The drawing under review shows one solid part. Ordinate dimensions are in mm from its lowest x, y, z. Give positions to 0.01 mm unless a question says otherwise; leave off trailing zeros. Order: outer loops, then holes, each group sorted by start corner. A loop starts at its lowest first (then second) coordinate and runs counter-clockwise, first axis right, second up. Notation, with made-up numbers: (22.25, 77) - (74.25, 77) arc R3 ccw to (74.25, 82) - close; hole circle Ø10 at (56.5, 61). An arc over 180 degrees is marked (long way). Use CSV: the item, a comma, the result in double quotes. Start each with the question number.
1. For pin 1 (2 mm diameter, centred on x = 86, y = 5, fed in from -Z); pin 2 (3 mm diameter, centred on x = 90, z = 9.5, fed in from -Y); pin 3 (8 mm diameter, centred on x = 62, z = 4, fed in from +Y), all flat-tipped, find the tip position at first contact; note any pin that passes through.
2. Take a section at C-C, the plane x = 7. State the section outline as (y, z) points.
3. Take a section at B-B, the plane z = 7. State the section outline as (x, y) points.
4. To check wall thickness, follow line 1 (X direction, y = 3, z = 7); line 2 (X direction, y = 4.5, z = 8.25); line 3 (Y direction, x = 43, z = 7). State the ranges of each line that lie inside material, in increasing order. Write a range as [from, to].
5. Take a section at A-A, the plane y = 3.5. State the section outline as (x, z) points.
6. Take a section at D-D, the plane x = 84. State the section outline as (y, z) points.
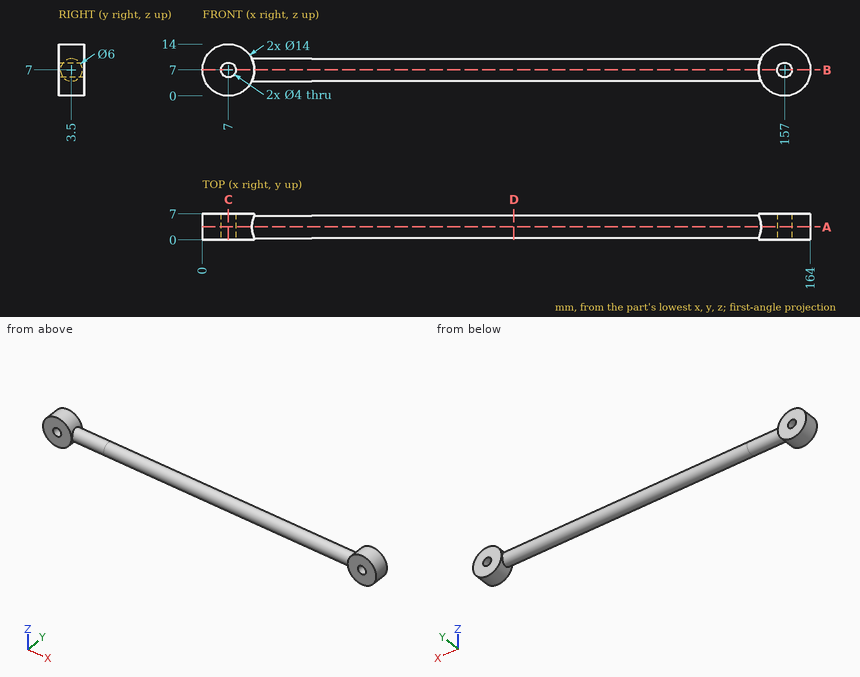
Determined:
1,pin 1,"stops at z = 4.04"
1,pin 2,"stops at y = 0.67"
1,pin 3,"stops at y = 6.5"
2,outline,"(0, 0) - (7, 0) - (7, 5) - (0, 5) - close; (0, 9) - (7, 9) - (7, 14) - (0, 14) - close"
3,outline,"(0, 0) - (5, 0) - (5, 7) - (0, 7) - close; (9, 0) - (14, 0) - (14, 0.5) - (150, 0.5) - (150, 0) - (155, 0) - (155, 7) - (150, 7) - (150, 6.5) - (14, 6.5) - (14, 7) - (9, 7) - close; (159, 0) - (164, 0) - (164, 7) - (159, 7) - close"
4,line 1,"x = [0, 5], [9, 155], [159, 164]"
4,line 2,"x = [0.11, 5.44], [8.56, 155.44], [158.56, 163.89]"
4,line 3,"y = [0.5, 6.5]"
5,outline,"(13.32, 4) - (150.68, 4) arc R7 ccw (long way) to (150.68, 10) - (13.32, 10) arc R7 ccw (long way) to start; hole circle Ø4 at (7, 7); hole circle Ø4 at (157, 7)"
6,outline,"circle Ø6 at (3.5, 7)"
